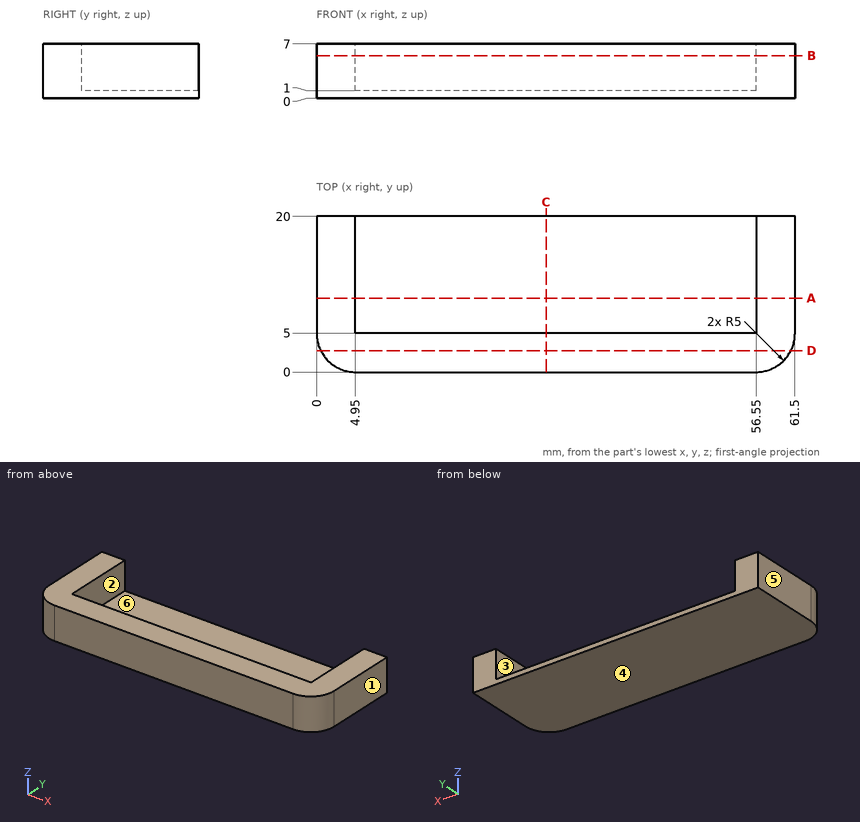
Here's the drawing with two shaded views (mm, measured from the low corner). I have some questions. A direction names the side the tool comes from. Coordinates: 2 decimals unless noted, no trailing zeros. Order: outer loops, then holes, each group sorted by start corner. A loop starts at its lowest first (then second) coordinate and runs counter-clockwise, first axis right, second up. Notation, with made-up numbers: (-25.5, 46) - (16.5, 46) arc R20 cw to (16.5, 68) - close; hole circle Ø9 at (-1.75, -33.75). An arc over 180 degrees is marked (long way). Answer in a Markdown table with one row per item. Add a question column.
(1) If we section it at A-A, the plane y = 9.5: Please give me the cut outline in (x, z).
(2) I need wall thicknesses on L1, parallel to X at y = 17, z = 2.5; L2, parallel to Z at x = 15.5, y = 18.75; L3, parallel to Y at x = 34.5, z = 1.5. Which ranges of each line are inside material? Lowest first, please.
(3) If we section it at B-B, the plane z = 5.5: Please give me the cut outline in (x, y), then the cut area to 3 significant figures.
(4) If we section it at C-C, the plane x = 29.5: Please give me the cut outline in (y, z), then the cut area to 3 significant figures.
(5) Will this pin go through, and if not, where does the flat tip stop? pin 1 (3 mm diameter, centred on x = 33, y = 16.5, fed in from +Z).
(6) On a 3-axis mill with a long thin cutter (end or side, diameter ignored), from which of +Z, -Z, +X, -X, +Y, -Y can I reach the whole of each face in a straight line? I mean the marked faces 5 and 6. Say none if no direction works.
(7) If we mould it in two halves opening along X, with no side actions, what happens to the marked faces 1, 2, 3 and 4? For each: released by +X, released by -X, zero draft, split by the parting line, or undercut.
(8) If we section it at D-D, the plane y = 2.75: Please give me the cut outline in (x, z), then the cut area to 3 significant figures.
Results are:
| question | item | result |
|---|---|---|
| 1 | outline | (0, 0) - (61.5, 0) - (61.5, 7) - (56.55, 7) - (56.55, 1) - (4.95, 1) - (4.95, 7) - (0, 7) - close |
| 2 | L1 | x = 0 to 4.95, 56.55 to 61.5 |
| 2 | L2 | z = 0 to 1 |
| 2 | L3 | y = 0 to 5 |
| 3 | outline | (0, 5) arc R5 ccw to (5, 0) - (56.5, 0) arc R5 ccw to (61.5, 5) - (61.5, 20) - (56.55, 20) - (56.55, 5) - (4.95, 5) - (4.95, 20) - (0, 20) - close |
| 3 | area | 445 mm2 |
| 4 | outline | (0, 0) - (20, 0) - (20, 1) - (5, 1) - (5, 7) - (0, 7) - close |
| 4 | area | 50.0 mm2 |
| 5 | pin 1 | stops at z = 1 |
| 6 | face 5 | +Z, -Z, -X, +Y, -Y |
| 6 | face 6 | +Z, +Y |
| 7 | face 1 | released by +X |
| 7 | face 2 | undercut |
| 7 | face 3 | undercut |
| 7 | face 4 | zero draft |
| 8 | outline | (0.53, 0) - (60.97, 0) - (60.97, 7) - (0.53, 7) - close |
| 8 | area | 423 mm2 |
